Read the model definition and answer for the solid it produces. Units are mm, in the model's axes. Face numbers are marked on the shaded views. A direction names the side the tool comes from. Coordinates: 2 decimals unless noted, no trailing zeros. Loops run counter-clockwise (first coordinate to the right, second up) from the corner with the lowest first, then second, coordinate; pieces in that order, holes last. Notation, with made-up numbers: M -29.5,88.5 L -12.5,88.5 A20 cw -12.5,116.5 Z; hole C 82,-21 d3. An arc over 180 degrees is marked long. Put each result on its own line as item: value.
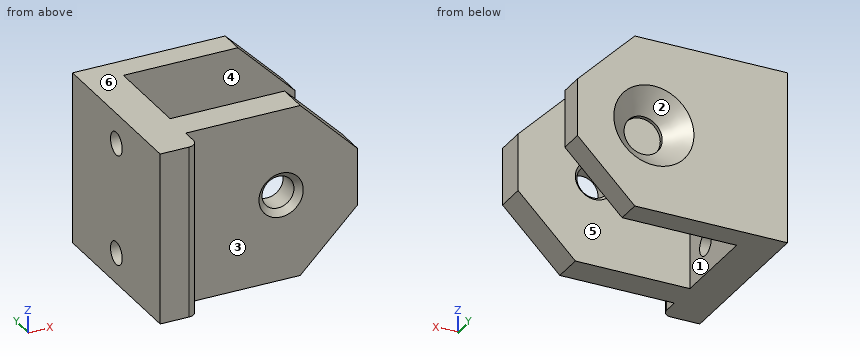
Autodesk Inventor part; units mm, degrees
ref_plane "bracket_to_screw_XY" through (35, 45, 0) normal (0, 1, 0) x (1, 0, 0)
ref_plane "bracket_to_screw_YZ" through (35, 45, 0) normal (1, 0, 0) x (0, 0, -1)
ref_plane "bracket_to_screw_ZX" through (35, 45, 0) normal (0, 0, -1) x (0, 1, 0)
sketch "Sketch_6" plane through (0, 0, 0) normal (0, 0, 1) x (1, 0, 0)
  line L0 (0, 45) -> (0, 0)
  line L1 (0, 0) -> (7.5, 0)
  arc A0 (7.5, 0) -> (10, 2.5) centre (7.5, 2.5) ccw
  line L2 (10, 2.5) -> (10, 6.5)
  line L3 (10, 6.5) -> (55, 6.5)
  line L4 (55, 6.5) -> (55, 14.5)
  line L5 (55, 14.5) -> (10, 14.5)
  line L6 (10, 14.5) -> (10, 38.5)
  line L7 (10, 38.5) -> (55, 38.5)
  line L8 (55, 38.5) -> (55, 45)
  line L9 (55, 45) -> (0, 45)
extrude "Extrusion1" add sketch "Sketch_6" along normal mid plane 45
sketch "Sketch_7" plane through (0, 0, 0) normal (0, 1, 0) x (-1, 0, 0)
  line L0 (-40, 22.5) -> (-110, 22.5)
  line L1 (-110, 22.5) -> (-110, -22.5)
  line L2 (-110, -22.5) -> (-40, -22.5)
  line L3 (-40, -22.5) -> (-55, -7.5)
  line L4 (-55, -7.5) -> (-55, 7.5)
  line L5 (-55, 7.5) -> (-40, 22.5)
extrude "Extrusion2" cut sketch "Sketch_7" along normal blind 45
sketch "Sketch_8" plane through (35, 0, 0) normal (1, 0, 0) x (0, 0, -1)
  line L0 (0, 6.5) -> (0, 14.5)
  line L1 (0, 14.5) -> (5, 14.5)
  line L2 (5, 14.5) -> (4.188, 13.688)
  line L3 (4.188, 13.688) -> (4.188, 8.112)
  line L4 (4.188, 8.112) -> (5.8, 6.5)
  line L5 (5.8, 6.5) -> (0, 6.5)
  line L6 (0, 6.5) -> (0, 14.5)
revolve "Revolution1" cut sketch "Sketch_8" angle 360 about axis through (35, 6.5, 0) along (0, -1, 0)
thread "Thread1"
sketch "Sketch4" plane through (0, 45, 22.5) normal (0, 1, 0) x (1, 0, 0)
  point P0 (35, 22.5)
hole "Hole1" at (35, 45, 0) direction (0, -1, 0) diameter 10 depth 6.5 countersink diameter 21 countersink angle 90
sketch "Sketch5" plane through (0, 0, 22.5) normal (-1, 0, 0) x (0, 0, 1)
  point P0 (-37, 22.5)
hole "Hole2" at (0, 22.5, -14.5) direction (1, 0, 0) diameter 6 depth 10
sketch "Sketch6" plane through (0, 0, 22.5) normal (-1, 0, 0) x (0, 0, 1)
  point P0 (-8, 22.5)
hole "Hole3" at (0, 22.5, 14.5) direction (1, 0, 0) diameter 6 depth 10
ref_plane "bracket_to_screw_XY" through (35, 45, 0) normal (0, 1, 0) x (1, 0, 0)
ref_plane "bracket_to_screw_YZ" through (35, 45, 0) normal (1, 0, 0) x (0, 0, -1)
ref_plane "bracket_to_screw_ZX" through (35, 45, 0) normal (0, 0, -1) x (0, 1, 0)
ref_plane "screw11_XY" through (10, 22.5, 14.5) normal (1, 0, 0) x (0, 0, -1)
ref_plane "screw11_YZ" through (10, 22.5, 14.5) normal (0, 0, -1) x (0, 1, 0)
ref_plane "screw11_ZX" through (10, 22.5, 14.5) normal (0, 1, 0) x (1, 0, 0)
ref_plane "screw12_XY" through (10, 22.5, -14.5) normal (1, 0, 0) x (0, 0, -1)
ref_plane "screw12_YZ" through (10, 22.5, -14.5) normal (0, 0, -1) x (0, 1, 0)
ref_plane "screw12_ZX" through (10, 22.5, -14.5) normal (0, 1, 0) x (1, 0, 0)
ref_plane "screw1_1_XY" through (-27.6, 22.5, 14.5) normal (-1, 0, 0) x (0, 0, -1)
ref_plane "screw1_1_YZ" through (-27.6, 22.5, 14.5) normal (0, 0, -1) x (0, -1, 0)
ref_plane "screw1_1_ZX" through (-27.6, 22.5, 14.5) normal (0, -1, 0) x (-1, 0, 0)
ref_plane "screw1_2_XY" through (-27.6, 22.5, -14.5) normal (-1, 0, 0) x (0, 0, -1)
ref_plane "screw1_2_YZ" through (-27.6, 22.5, -14.5) normal (0, 0, -1) x (0, -1, 0)
ref_plane "screw1_2_ZX" through (-27.6, 22.5, -14.5) normal (0, -1, 0) x (-1, 0, 0)
ref_plane "screw2_XY" through (10, 22.5, 0) normal (1, 0, 0) x (0, 0, -1)
ref_plane "screw2_YZ" through (10, 22.5, 0) normal (0, 0, -1) x (0, 1, 0)
ref_plane "screw2_ZX" through (10, 22.5, 0) normal (0, 1, 0) x (1, 0, 0)
ref_plane "screw22_XY" through (2.2, 22.5, 0) normal (1, 0, 0) x (0, 0, -1)
ref_plane "screw22_YZ" through (2.2, 22.5, 0) normal (0, 0, -1) x (0, 1, 0)
ref_plane "screw22_ZX" through (2.2, 22.5, 0) normal (0, 1, 0) x (1, 0, 0)
ref_plane "screw3_XY" through (0, 22.5, 14.5) normal (1, 0, 0) x (0, 0, -1)
ref_plane "screw3_YZ" through (0, 22.5, 14.5) normal (0, 0, -1) x (0, 1, 0)
ref_plane "screw3_ZX" through (0, 22.5, 14.5) normal (0, 1, 0) x (1, 0, 0)
ref_plane "screw3_1_XY" through (0, 22.5, -14.5) normal (1, 0, 0) x (0, 0, -1)
ref_plane "screw3_1_YZ" through (0, 22.5, -14.5) normal (0, 0, -1) x (0, 1, 0)
ref_plane "screw3_1_ZX" through (0, 22.5, -14.5) normal (0, 1, 0) x (1, 0, 0)
properties part number "HBLTBBN45-SET_b"
1) Find section C-C, the plane y = 22.5. Write down the section's boundary in (x, z), plus the area to 3 significant figures.
Answer list:
outline: M 0,-22.5 L 10,-22.5 L 10,-17.5 L 0,-17.5 Z; M 0,-11.5 L 10,-11.5 L 10,11.5 L 0,11.5 Z; M 0,17.5 L 10,17.5 L 10,22.5 L 0,22.5 Z
area: 330 mm^2
2) Which of the six approach directions +Z, -Z, +X, -X, +Y, -Y give full straight-line access (tool end or side, diameter ignored) to the marked faces 5 and 6?
Answer list:
face 5: +Z, -Z, +X
face 6: +Z, +X, -X, +Y, -Y
3) Straight lines are drawn through the part: line 1 (Y direction, x = 49, z = -1); line 2 (Z direction, x = 7.5, y = 22.5); line 3 (X direction, y = 10.95, z = 0). For each, find the intervals that lie inside material, in ascending order. Write a range as [from, to].
Answer list:
line 1: y = [6.5, 14.5], [38.5, 45]
line 2: z = [-22.5, -17.5], [-11.5, 11.5], [17.5, 22.5]
line 3: x = [0, 30.81], [39.19, 55]
4) Find section A-A, the plane z = 0. Write down the section's boundary in (x, y), plus the area to 3 significant figures.
Answer list:
outline: M 0,0 L 7.5,0 A2.5 ccw 10,2.5 L 10,6.5 L 29.2,6.5 L 30.81,8.11 L 30.81,13.69 L 30,14.5 L 10,14.5 L 10,38.5 L 30,38.5 L 30,39.5 L 24.5,45 L 0,45 Z; M 39.19,8.11 L 40.8,6.5 L 55,6.5 L 55,14.5 L 40,14.5 L 39.19,13.69 Z; M 40,38.5 L 55,38.5 L 55,45 L 45.5,45 L 40,39.5 Z
area: 936 mm^2
5) Find section D-D, the plane z = 14.5. Write down the section's boundary in (x, y).
Answer list:
outline: M 0,0 L 7.5,0 A2.5 ccw 10,2.5 L 10,6.5 L 48,6.5 L 48,14.5 L 10,14.5 L 10,19.5 L 0,19.5 Z; M 0,25.5 L 10,25.5 L 10,38.5 L 48,38.5 L 48,45 L 0,45 Z
6) Find section B-B, the plane x = 35. Write down the section's boundary in (y, z).
Answer list:
outline: M 6.5,-22.5 L 14.5,-22.5 L 14.5,-5 L 13.69,-4.19 L 8.11,-4.19 L 6.5,-5.8 Z; M 6.5,5.8 L 8.11,4.19 L 13.69,4.19 L 14.5,5 L 14.5,22.5 L 6.5,22.5 Z; M 38.5,-22.5 L 45,-22.5 L 45,-10.5 L 39.5,-5 L 38.5,-5 Z; M 38.5,5 L 39.5,5 L 45,10.5 L 45,22.5 L 38.5,22.5 Z
7) Determine the mould class of the marked faces 1, 2, 3 and 4 for opening direction Y: released by +Y, released by -Y, zero draft, split by the parting line, or undercut.
Answer list:
face 1: undercut
face 2: released by +Y
face 3: released by -Y
face 4: undercut
8) Given pin 1 Ø12 at (y, z) = (31.5, -2) entering from +X; pin 2 Ø1 at (x, z) = (38, 16.5) entering from -Y; pin 3 Ø9 at (x, z) = (35, 0) entering from -Y, each flat-ended and moving along its own axis, determine where each tip first touches the part or whether it passes through.
Answer list:
pin 1: stops at x = 10
pin 2: stops at y = 6.5
pin 3: stops at y = 7.8
